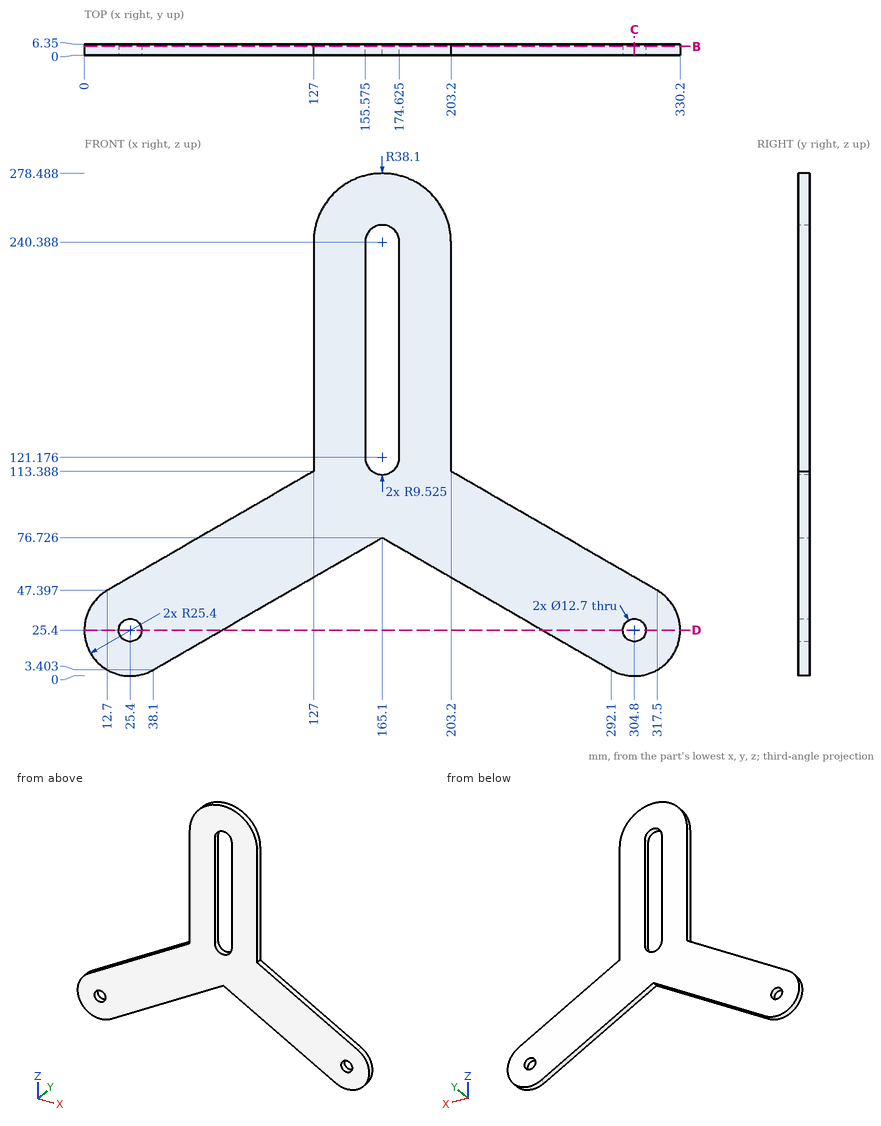
For this review, use the dimensioned drawing (mm, ordinates from the lowest corner) and the shaded views. Give positions to 0.01 mm unless a question says otherwise; leave off trailing zeros. Write each loop counter-clockwise with the first axis right and the second up, starting at its lowest first coordinate (ties: lowest second). Pieces come first, ordered by that corner, then holes. Notation, with made-up numbers: M 53,37.25 L 94,37.25 A16 ccw 94,59.25 Z; hole C -26.75,21.5 d4. An arc over 180 degrees is marked long. Answer as a JSON object with one key per item and string values. Group by question number.
Item 1: For probe 1 along X at (y, z) = (2.25, 207) (1 decimal); probe 2 along X at (y, z) = (3.5, 25.4); probe 3 along X at (y, z) = (4.75, 114) (1 decimal), list the stretches that pass through material, from the lowest coordinate up. Write a range as [from, to].
Item 2: Consider section D-D on z = 25.4. Write out the cut boundary in (x, y).
Item 3: For pin 1 Ø1.9 at (y, z) = (2.5, 194.5) entering from +X; pin 2 Ø1.5 at (x, y) = (208.5, 2) entering from -Z; pin 3 Ø2 at (x, y) = (294, 1.5) entering from +Z, all flat-tipped, find the tip position at first contact; note any pin that passes through.
Item 4: Consider section B-B on y = 5. Count the separate pieces of the cut face and the enclosed holes in it, plus the area to 3 significant figures.
Item 5: Consider section C-C on x = 304.8. Write out the cut boundary in (y, z).
Check result:
{
 "1": {"probe 1": "x = [127, 155.6], [174.6, 203.2]", "probe 2": "x = [0, 19.05], [31.75, 76.2], [254, 298.45], [311.15, 330.2]", "probe 3": "x = [127, 158.8], [171.4, 203.2]"},
 "2": {"outline": "M 0,0 L 19.05,0 L 19.05,6.35 L 0,6.35 Z; M 31.75,0 L 76.2,0 L 76.2,6.35 L 31.75,6.35 Z; M 254,0 L 298.45,0 L 298.45,6.35 L 254,6.35 Z; M 311.15,0 L 330.2,0 L 330.2,6.35 L 311.15,6.35 Z"},
 "3": {"pin 1": "stops at x = 203.2", "pin 2": "stops at z = 51.24", "pin 3": "stops at z = 61.54"},
 "4": {"separate pieces": "1", "enclosed holes": "3", "area": "26,700 mm^2"},
 "5": {"outline": "M 0,0 L 6.35,0 L 6.35,19.05 L 0,19.05 Z; M 0,31.75 L 6.35,31.75 L 6.35,54.73 L 0,54.73 Z"}
}
